```python
from build123d import *

# Parameters (mm, degrees)
BOSS_EXTRUDE1_DEPTH = 100


with BuildPart() as part:
    # Sketch1 → Boss-Extrude1 (new body)
    with BuildSketch(Plane(origin=(0, 0, 0), x_dir=(1, 0, 0), z_dir=(0, 1, 0))):
        with BuildLine():
            Line((-135.351509673, -54.659892728), (-143.16186287, 28.502913245))
            ThreePointArc((-143.16186287, 28.502913245), (-142.333418361, 32.387236089), (-141.399603301, 36.247582406))
            Line((-141.399603301, 36.247582406), (-70.729724798, 127.691194191))
            ThreePointArc((-70.729724798, 127.691194191), (1.701551679, 145.961775016), (73.687223064, 126.007651359))
            ThreePointArc((73.687223064, 126.007651359), (111.65776791, 66.863352087), (145.869241729, 5.468030837))
            ThreePointArc((145.869241729, 5.468030837), (125.636702297, -60.683640158), (86.399335375, -117.655811121))
            ThreePointArc((86.399335375, -117.655811121), (18.367849273, -132.71304327), (-51.195880989, -136.699366544))
            ThreePointArc((-51.195880989, -136.699366544), (-98.238828154, -100.772834831), (-135.351509673, -54.659892728))
        make_face()
    extrude(amount=BOSS_EXTRUDE1_DEPTH)


solid = part.part
```
The listing builds one solid part. Answer for the finished solid, in the listing's coordinates (mm). Give positions to 0.01 mm unless a question says otherwise; leave off trailing zeros. Write each loop counter-clockwise with the first axis right and the second up, starting at its lowest first coordinate (ties: lowest second). Pieces come first, ordered by that corner, then holes. Notation, with made-up numbers: (-26, 28) - (32, 28) arc R18 cw to (32, 48) - close; hole circle Ø8 at (13.5, 48.5). An arc over 180 degrees is marked (long way). Use one line per item in the form item = value. Start each with the question number.
1) Find section A-A on y = 47.5. Determine the outline of the cut face in (x, z), plus the area to 3 significant figures.
2) Flat-ended cylindrical pins translate along their axes: pin 1 Ø5 at (x, y) = (75, 23.5) entering from -Z; pin 2 Ø8 at (y, z) = (22, 91) entering from +X; pin 3 Ø1.5 at (x, y) = (-78.5, 37) entering from +Z. Find the tip coordinate at first contact, or state that the pin passes through.
3) Consider line 1 along Z through (x, y) = (-83.5, 35); line 2 along Z through (x, y) = (-79.5, 92.5); line 3 along X through (y, z) = (45.5, -83.5). Determine where each line is inside the solid, lowest interval first. Write a range as from..to.
4) Find section C-C on x = -92. Determine the outline of the cut face in (y, z), plus the area to 3 significant figures.
5) Find section B-B on z = 65. Determine the outline of the cut face in (x, y) (3 decimals), plus the area to 3 significant figures.
Geometry results:
q1.outline = (-143.16, -28.5) arc R145.97 ccw to (-141.4, -36.25) - (-70.73, -127.69) arc R145.97 ccw to (73.69, -126.01) arc R1127.42 ccw to (145.87, -5.47) arc R226.74 ccw to (86.4, 117.66) arc R434.4 ccw to (-51.2, 136.7) arc R246.3 ccw to (-135.35, 54.66) - close
q1.area = 62,000 mm2
q2.pin_1 = -126.69
q2.pin_2 = 110.68
q2.pin_3 = 118.65
q3.line_1 = -111.17..114.03
q3.line_2 = -116.34..117.27
q3.line_3 = -104.88..101.5
q4.outline = (0, -100.17) - (100, -100.17) - (100, 106.65) - (0, 106.65) - close
q4.area = 20,700 mm2
q5.outline = (-128.542, 0) - (123.495, 0) - (123.495, 100) - (-128.542, 100) - close
q5.area = 25,200 mm2
